Could you check a few things on this drawing? It's one solid part, dimensions in mm from its lowest x, y, z. Coordinates: 2 decimals unless noted, no trailing zeros. Loops run counter-clockwise (first coordinate to the right, second up) from the corner with the lowest first, then second, coordinate; pieces in that order, holes last. Notation, with made-up numbers: M -17.75,-31 L 9.25,-31 A16 ccw 9.25,-12 Z; hole C 11.25,28.5 d9. An arc over 180 degrees is marked long. Use one line per item in the form item = value. Start each with the question number.
(1) Will these pins go through, and if not, where does the flat tip stop? P1, Ø13, axis at x = 353.24, z = 163.37, coming from the +Y side; P2, Ø1, axis at x = 91.5, y = 1.5, coming from the -Z side.
(2) Imagine slicing it at B-B, the plane y = 1.4. Please give me the cut outline in (x, z) (1 decimal).
(3) Imagine slicing it at D-D, the plane x = 339.5. Please give me the cut outline in (y, z) (1 decimal).
(4) Please list where these lines run through material, in increasing order: L1, parallel to Z at x = 166, y = 2.2 (1 decimal); L2, parallel to X at y = 1.5, z = 71.5 (1 decimal); L3, parallel to Z at x = 106, y = 1.4 (1 decimal).
(5) Imagine slicing it at C-C, the plane z = 119. Please give me the cut outline in (x, y) (1 decimal).
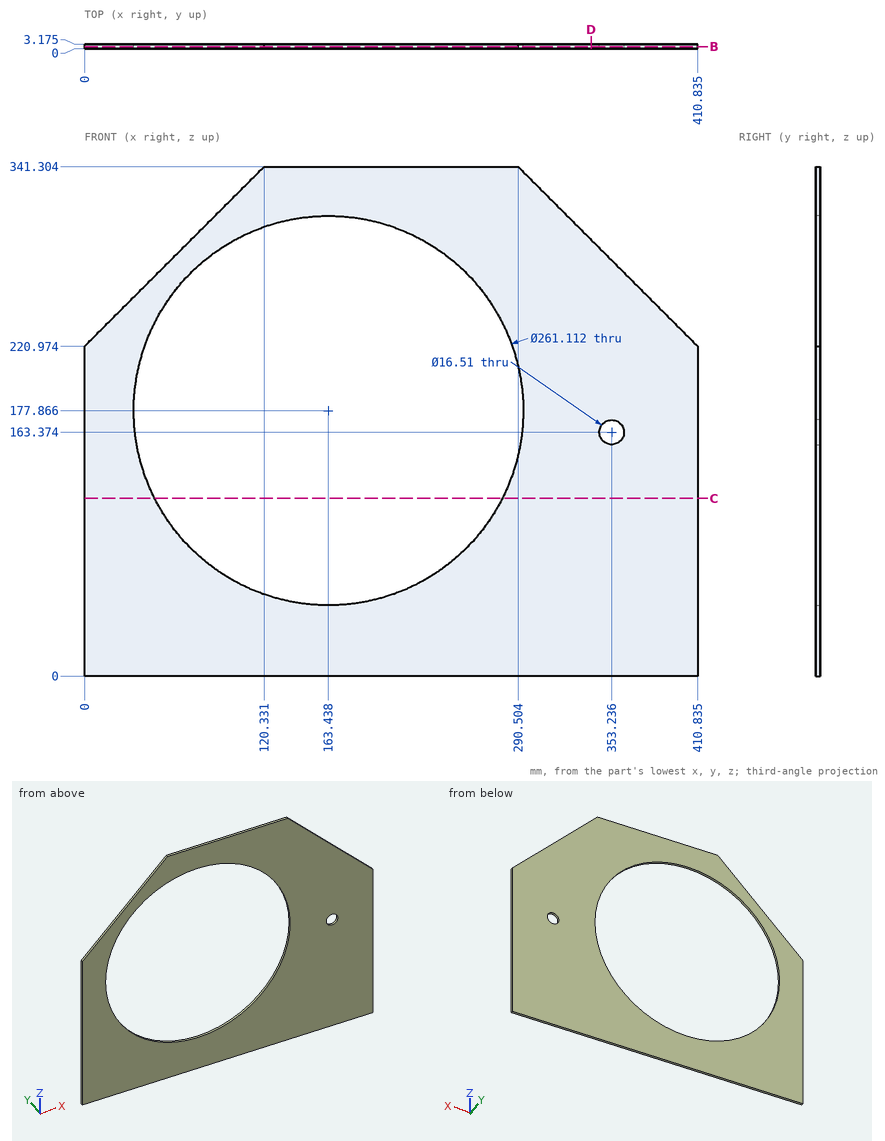
Answer:
q1.P1 = through
q1.P2 = 0
q2.outline = M 0,0 L 410.8,0 L 410.8,221 L 290.5,341.3 L 120.3,341.3 L 0,221 Z; hole C 163.4,177.9 d261.1; hole C 353.2,163.4 d16.5
q3.outline = M 0,0 L 3.2,0 L 3.2,292.3 L 0,292.3 Z
q4.L1 = 0 to 47.3, 308.4 to 341.3
q4.L2 = 0 to 87.7, 239.1 to 410.8
q4.L3 = 0 to 60.6, 295.1 to 327
q5.outline = M 0,0 L 46.9,0 L 46.9,3.2 L 0,3.2 Z; M 280,0 L 410.8,0 L 410.8,3.2 L 280,3.2 Z
